from build123d import *

# Parameters (mm, degrees)
F0_W     = 50.8
F0_H     = 38.1
F1_DEPTH = 29.21
F2_R     = 2.54
F3_R     = 6.35
F4_DEPTH = 50.8


with BuildPart() as f1:
    # F0 (on Front) → F1 (new body)
    with BuildSketch(Plane.XZ):
        with Locations((-25.4, -19.05)):
            Rectangle(F0_W, F0_H)
    extrude(amount=F1_DEPTH)

    # F2
    f2_edges = [f1.edges().sort_by_distance(p)[0] for p in [
        (-25.4, -29.21, 0),
    ]]
    fillet(f2_edges, radius=F2_R)

    # F3 (on face) → F4 (cut, through all)
    with BuildSketch(Plane.YZ):
        with Locations((-12.7, -15.24)):
            Circle(F3_R)
    extrude(amount=-F4_DEPTH, mode=Mode.SUBTRACT)


solid = f1.part
The model under review builds one solid part; all positions refer to its coordinate system, in mm. Give positions to 0.01 mm unless a question says otherwise; leave off trailing zeros. Loops run counter-clockwise (first coordinate to the right, second up) from the corner with the lowest first, then second, coordinate; pieces in that order, holes last. Notation, with made-up numbers: (39.5, -35) -> (59.5, -35) arc R10 cw to (59.5, -31) -> close; hole circle Ø5 at (16.5, 83.25). An arc over 180 degrees is marked (long way). Put each result on its own line as item: value. Start each with the question number.
1. Wall thickness on probe 1 along Z at (x, y) = (-33, -9.5); probe 2 along Z at (x, y) = (-42, -13.75); probe 3 along Y at (x, z) = (-37.5, -16.5): over which ranges is each line inside the solid? List them lowest first.
2. We need section A-A on y = -12.7. State the section outline as (x, z) points, then the cut area to 3 significant figures.
3. We need section B-B on z = -15.24. State the section outline as (x, y) points, then the cut area to 3 significant figures.
4. We need section C-C on x = -15. State the section outline as (y, z) points.
5. Mouldability with a two-part tool opening along Z and no side actions: class faces 1 (the face through (-25.044, -6.643, -13.333)), 2 (the face through (0, -14, -24)), 3 (the face through (-25.044, -28.446, -0.724)) as released by +Z, released by -Z, zero draft, split by the parting line, or undercut.
Determined:
1. probe 1: -38.1 to -20.72, -9.76 to 0
1. probe 2: -38.1 to -21.5, -8.98 to 0
1. probe 3: -29.21 to -18.92, -6.48 to 0
2. outline: (-50.8, -38.1) -> (0, -38.1) -> (0, -21.59) -> (-50.8, -21.59) -> close; (-50.8, -8.89) -> (0, -8.89) -> (0, 0) -> (-50.8, 0) -> close
2. area: 1,290 mm^2
3. outline: (-50.8, -29.21) -> (0, -29.21) -> (0, -19.05) -> (-50.8, -19.05) -> close; (-50.8, -6.35) -> (0, -6.35) -> (0, 0) -> (-50.8, 0) -> close
3. area: 839 mm^2
4. outline: (-29.21, -38.1) -> (0, -38.1) -> (0, 0) -> (-26.67, 0) arc R2.54 ccw to (-29.21, -2.54) -> close; hole circle Ø12.7 at (-12.7, -15.24)
5. face 1: undercut
5. face 2: zero draft
5. face 3: released by +Z
